```python
from build123d import *

# Parameters (mm, degrees)
CYLINDER_R        = 0.3
CYLINDER_DEPTH    = 11
CYLINDER001_R     = 0.3
CYLINDER001_DEPTH = 11
CYLINDER002_R     = 0.3
CYLINDER002_DEPTH = 11
CYLINDER003_R     = 0.3
CYLINDER003_DEPTH = 11
SKETCH_W          = 27.5
SKETCH_H          = 27.5
PAD_DEPTH         = 1.1
SKETCH001_R       = 1
POCKET_DEPTH      = 1.1
PAD001_DEPTH      = 2.1


with BuildPart() as zylinder:
    # Cylinder → Cylinder (new body)
    with BuildSketch(Plane(origin=(-3.81, 11, -8.5), x_dir=(1, 0, 0), z_dir=(0, 0, 1))):
        Circle(CYLINDER_R)
    extrude(amount=CYLINDER_DEPTH)


with BuildPart() as zylinder001:
    # Cylinder001 → Cylinder001 (new body)
    with BuildSketch(Plane(origin=(-1.27, 11, -8.5), x_dir=(1, 0, 0), z_dir=(0, 0, 1))):
        Circle(CYLINDER001_R)
    extrude(amount=CYLINDER001_DEPTH)


with BuildPart() as zylinder002:
    # Cylinder002 → Cylinder002 (new body)
    with BuildSketch(Plane(origin=(3.81, 11, -8.5), x_dir=(1, 0, 0), z_dir=(0, 0, 1))):
        Circle(CYLINDER002_R)
    extrude(amount=CYLINDER002_DEPTH)


with BuildPart() as zylinder003:
    # Cylinder003 → Cylinder003 (new body)
    with BuildSketch(Plane(origin=(1.27, 11, -8.5), x_dir=(1, 0, 0), z_dir=(0, 0, 1))):
        Circle(CYLINDER003_R)
    extrude(amount=CYLINDER003_DEPTH)


with BuildPart() as fusion:
    # Sketch → Pad (new body)
    with BuildSketch(Plane.XY):
        Rectangle(SKETCH_W, SKETCH_H)
    extrude(amount=PAD_DEPTH)

    # Sketch001 → Pocket (cut)
    with BuildSketch(Plane.XY):
        with Locations((-11.5, 11.5)):
            Circle(SKETCH001_R)
        with Locations((11.5, 11.5)):
            Circle(SKETCH001_R)
        with Locations((11.5, -11.5)):
            Circle(SKETCH001_R)
        with Locations((-11.5, -11.5)):
            Circle(SKETCH001_R)
    extrude(amount=POCKET_DEPTH, mode=Mode.SUBTRACT)

    # Sketch002 (on Face5 of Pocket) → Pad001 (join)
    with BuildSketch(Plane.XY.offset(1.1)):
        Polygon((-13.75, 9.75), (13.75, 9.75), (13.75, -9.25), (6, -9.25), (6, -13.75), (-6, -13.75), (-6, -9.25), (-13.75, -9.25), align=None)
    extrude(amount=PAD001_DEPTH)

    # Fusion: union Zylinder, Zylinder001, Zylinder002, Zylinder003
    add(zylinder.part)
    add(zylinder001.part)
    add(zylinder002.part)
    add(zylinder003.part)


solid = fusion.part
```
Geometry: final body of the model. Coordinates: model frame, mm. A direction names the side the tool comes from. Round coordinates to 2 decimals unless told otherwise and drop trailing zeros. Loops run counter-clockwise (first coordinate to the right, second up) from the corner with the lowest first, then second, coordinate; pieces in that order, holes last.
Item 1: Section C-C, the plane y = 4.5. Output: boundary loops of the cut face in (x, z).
Checked values:
outline: (-13.75, 0) - (13.75, 0) - (13.75, 3.2) - (-13.75, 3.2) - close
Item 2: Section B-B, the plane z = -7.25. Output: boundary loops of the cut face in (x, y), plus the area to 3 significant figures.
Checked values:
outline: circle Ø0.6 at (-3.81, 11); circle Ø0.6 at (-1.27, 11); circle Ø0.6 at (1.27, 11); circle Ø0.6 at (3.81, 11)
area: 1.13 mm2
Item 3: Reachability of faces 1 (the flat face through (-10, -9.25, 2)), 2 (the flat face through (10, -9.25, 2)), 3 (the cylindrical face through (10.7, 10.9, 0.5)) from +Z, -Z, +X, -X, +Y, -Y: full face, straight path, thin tool, end or side. Return the list, or none.
Checked values:
face 1: +Z, -X, -Y
face 2: +Z, +X, -Y
face 3: +Z, -Z
Item 4: Line query: L1, parallel to Y at x = -11.5, z = 0.4; L2, parallel to Y at x = 12.5, z = 2.25; L3, parallel to Z at x = -4, y = -10.75. Output: solid intervals per line, ascending.
Checked values:
L1: y = -13.75 to -12.5, -10.5 to 10.5, 12.5 to 13.75
L2: y = -9.25 to 9.75
L3: z = 0 to 3.2
Item 5: Contact query for flat-ended pins moving along their axis: P1, Ø1.2, axis at x = 3, y = 12.5, coming from the +Z side; P2, Ø0.7, axis at x = -3.5, y = 11, coming from the +Z side; P3, Ø1.5, axis at x = -5, z = -6, coming from the -Y side; P4, Ø0.6, axis at x = -2.5, z = 2.5, coming from the +Y side. Output: stop coordinate, or through.
Checked values:
P1: stops at z = 1.1
P2: stops at z = 2.5
P3: passes through
P4: stops at y = 9.75
Item 6: Section D-D, the plane x = 11. Output: boundary loops of the cut face in (y, z).
Checked values:
outline: (-13.75, 0) - (-12.37, 0) - (-12.37, 1.1) - (-13.75, 1.1) - close; (-10.63, 0) - (10.63, 0) - (10.63, 1.1) - (9.75, 1.1) - (9.75, 3.2) - (-9.25, 3.2) - (-9.25, 1.1) - (-10.63, 1.1) - close; (12.37, 0) - (13.75, 0) - (13.75, 1.1) - (12.37, 1.1) - close
Item 7: Section A-A, the plane x = -11.5. Output: boundary loops of the cut face in (y, z).
Checked values:
outline: (-13.75, 0) - (-12.5, 0) - (-12.5, 1.1) - (-13.75, 1.1) - close; (-10.5, 0) - (10.5, 0) - (10.5, 1.1) - (9.75, 1.1) - (9.75, 3.2) - (-9.25, 3.2) - (-9.25, 1.1) - (-10.5, 1.1) - close; (12.5, 0) - (13.75, 0) - (13.75, 1.1) - (12.5, 1.1) - close
